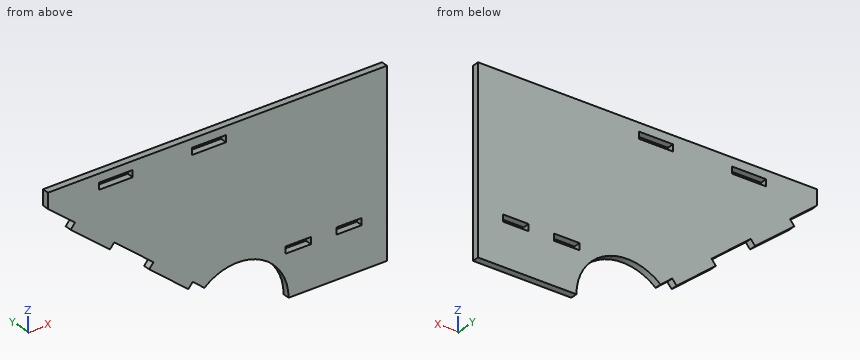
from build123d import *

# Parameters (mm, degrees)
SKETCH1_W           = 200
SKETCH1_H           = 108
BOSS_EXTRUDE1_DEPTH = 4
CUT_EXTRUDE1_DEPTH  = 228.332355814
SKETCH4_W           = 30
SKETCH4_H           = 4
BOSS_EXTRUDE2_DEPTH = 4
SKETCH5_W           = 15
SKETCH5_H           = 4
SKETCH5_W_2         = 20
CUT_EXTRUDE2_DEPTH  = 228.332355814
SKETCH6_R           = 30.118776273
CUT_EXTRUDE4_DEPTH  = 228.332355814


with BuildPart() as part:
    # Sketch1 → Boss-Extrude1 (new body)
    with BuildSketch(Plane(origin=(0, 0, 0), x_dir=(1, 0, 0), z_dir=(0, 1, 0))):
        with Locations((100, 54)):
            Rectangle(SKETCH1_W, SKETCH1_H)
    extrude(amount=BOSS_EXTRUDE1_DEPTH)

    # Sketch3 → Cut-Extrude1 (cut, through all)
    with BuildSketch(Plane(origin=(0, 4, 0), x_dir=(1, 0, 0), z_dir=(0, 1, 0))):
        Polygon((120.09925776, 108), (0, 9), (0, 108), align=None)
    extrude(amount=-CUT_EXTRUDE1_DEPTH, mode=Mode.SUBTRACT)

    # Sketch4 → Boss-Extrude2 (add)
    with BuildSketch(Plane(origin=(-4.417303696, 0, -5.358736315), x_dir=(-0.7716314833522663, 0, 0.6360698498589453), z_dir=(-0.6360698498589453, 0, -0.7716314833522663))):
        with Locations((-101.3679122, 2)):
            Rectangle(SKETCH4_W, SKETCH4_H)
        with Locations((-41.3679122, 2)):
            Rectangle(SKETCH4_W, SKETCH4_H)
    extrude(amount=BOSS_EXTRUDE2_DEPTH)

    # Sketch5 → Cut-Extrude2 (cut, through all)
    with BuildSketch(Plane(origin=(0, 4, 0), x_dir=(1, 0, 0), z_dir=(0, 1, 0))):
        with Locations((177.594068765, 80.999936793)):
            Rectangle(SKETCH5_W, SKETCH5_H)
        with Locations((147.594068765, 80.999936793)):
            Rectangle(SKETCH5_W, SKETCH5_H)
        with Locations((95, 7)):
            Rectangle(SKETCH5_W_2, SKETCH5_H)
        with Locations((40, 7)):
            Rectangle(SKETCH5_W_2, SKETCH5_H)
    extrude(amount=-CUT_EXTRUDE2_DEPTH, mode=Mode.SUBTRACT)

    # Sketch6 → Cut-Extrude4 (cut, through all)
    with BuildSketch(Plane(origin=(0, 4, 0), x_dir=(1, 0, 0), z_dir=(0, 1, 0))):
        with Locations((111.819464, 108)):
            Circle(SKETCH6_R)
    extrude(amount=-CUT_EXTRUDE4_DEPTH, mode=Mode.SUBTRACT)


solid = part.part
Check sheet for the modelled part. Datum: model origin and axes. Units: mm. Give positions to 0.01 mm unless a question says otherwise; leave off trailing zeros. Order: outer loops, then holes, each group sorted by start corner. A loop starts at its lowest first (then second) coordinate and runs counter-clockwise, first axis right, second up. Notation, with made-up numbers: M 34.5,31.5 L 89.5,31.5 A18 ccw 89.5,60.5 Z; hole C 0.5,75 d7. An arc over 180 degrees is marked long. Answer as CSV lines item,"result". Start each with the question number.
Item 1: Gauge pin test, flat ends, axial feed: P1, Ø1.2, axis at x = 177.5, y = 3, coming from the +Z side; P2, Ø2, axis at y = 3, z = -89, coming from the -X side; P3, Ø1.5, axis at x = 80, y = 1.5, coming from the -Z side; P4, Ø2, axis at y = 1, z = -80.5, coming from the -X side. Record the tip position at first contact, or that the pin passes through.
Item 2: Cross-section at A-A on y = 1.1. State how many separate pieces and enclosed holes the cut face has, plus the area to 3 significant figures.
Item 3: Cross-section at B-B on x = 32. Enter the section's corners in (y, z), plus the area to 3 significant figures.
Item 4: Thickness scan on line 1 (Z direction, x = 146, y = 1.9); line 2 (Z direction, x = 93, y = 1); line 3 (Z direction, x = 29.5, y = 1.85). Record the ranges inside material, lowest first. Write a range as [from, to].
Item 5: Cross-section at D-D on x = 113. Enter the section's corners in (y, z), plus the area to 3 significant figures.
Item 6: Cross-section at C-C on z = -37.5. Enter the section's corners in (x, y), plus the area to 3 significant figures.
Established:
1,P1,"stops at z = 0"
1,P2,"stops at x = 134.34"
1,P3,"stops at z = -80.75"
1,P4,"stops at x = 79.24"
2,separate pieces,"1"
2,enclosed holes,"4"
2,area,"14,700 mm^2"
3,outline,"M 0,-40.56 L 4,-40.56 L 4,-9 L 0,-9 Z; M 0,-5 L 4,-5 L 4,0 L 0,0 Z"
3,area,"146 mm^2"
4,line 1,"z = [-108, -83], [-79, 0]"
4,line 2,"z = [-84.48, -9], [-5, 0]"
4,line 3,"z = [-38.5, 0]"
5,outline,"M 0,-77.9 L 4,-77.9 L 4,0 L 0,0 Z"
5,area,"312 mm^2"
6,outline,"M 28.29,0 L 200,0 L 200,4 L 28.29,4 Z"
6,area,"687 mm^2"
